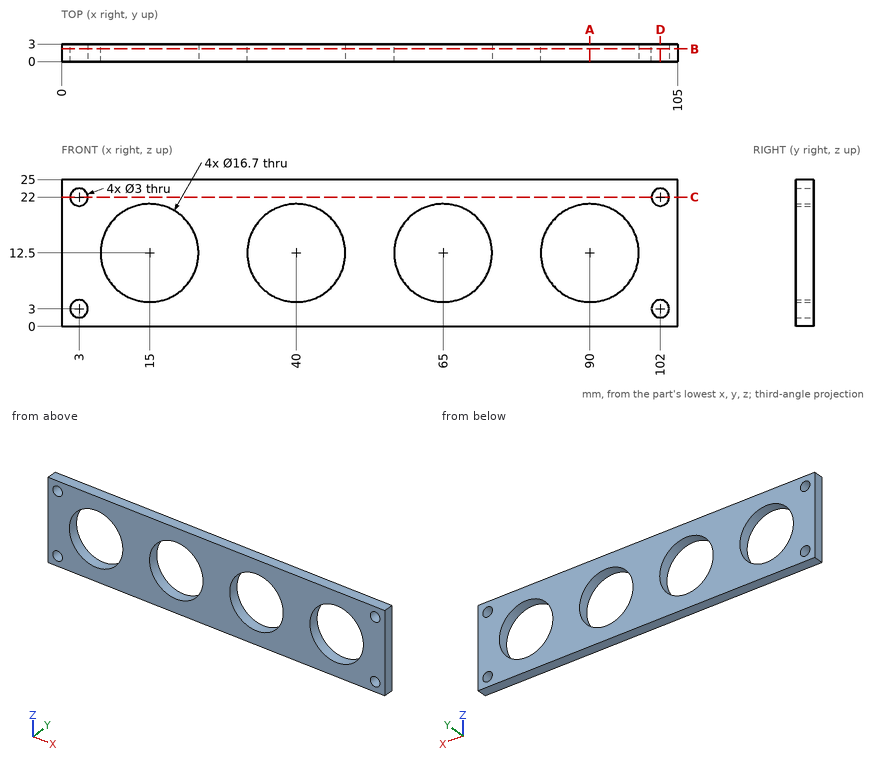
The drawing under review shows one solid part. Ordinate dimensions are in mm from its lowest x, y, z. Round coordinates to 2 decimals unless told otherwise and drop trailing zeros. Write each loop counter-clockwise with the first axis right and the second up, starting at its lowest first coordinate (ties: lowest second). Pieces come first, ordered by that corner, then holes. Notation, with made-up numbers: (4, 56) -> (28, 56) arc R8 cw to (28, 71) -> close; hole circle Ø7 at (67.25, 24). An arc over 180 degrees is marked (long way). One line per question, with ' | ' between items.
(1) Take a section at C-C, the plane z = 22. State the section outline as (x, y) points.
Result sheet:
outline: (0, 0) -> (1.5, 0) -> (1.5, 3) -> (0, 3) -> close; (4.5, 0) -> (100.5, 0) -> (100.5, 3) -> (4.5, 3) -> close; (103.5, 0) -> (105, 0) -> (105, 3) -> (103.5, 3) -> close
(2) Take a section at D-D, the plane x = 102. State the section outline as (y, z) points, and give its area (3 significant figures).
Result sheet:
outline: (0, 0) -> (3, 0) -> (3, 1.5) -> (0, 1.5) -> close; (0, 4.5) -> (3, 4.5) -> (3, 20.5) -> (0, 20.5) -> close; (0, 23.5) -> (3, 23.5) -> (3, 25) -> (0, 25) -> close | area: 57.0 mm2
(3) Insertion check: P1, Ø4, axis at x = 51.5, z = 7, coming from the -Y side; P2, Ø13.5, axis at x = 15, z = 12.5, coming from the +Y side. Each pin has a flat end and moves straight along its axis. Give the tip position at first contact, or say it passes through.
Result sheet:
P1: y = 0 | P2: through
(4) Take a section at B-B, the plane y = 2.15. State how many separate pieces and enclosed holes the cut face has, and give its area (3 significant figures).
Result sheet:
separate pieces: 1 | enclosed holes: 8 | area: 1,720 mm2
(5) Wall thickness on line 1 (X direction, y = 1.95, z = 2.75); line 2 (Z direction, x = 90, y = 2.2); line 3 (X direction, y = 1.6, z = 9.25): over which ranges is each line inside the solid? List them lowest first. Write a range as [from, to].
Result sheet:
line 1: [0, 1.52], [4.48, 100.52], [103.48, 105] | line 2: [0, 4.15], [20.85, 25] | line 3: [0, 7.31], [22.69, 32.31], [47.69, 57.31], [72.69, 82.31], [97.69, 105]
(6) Take a section at A-A, the plane x = 90. State the section outline as (y, z) points, and give its area (3 significant figures).
Result sheet:
outline: (0, 0) -> (3, 0) -> (3, 4.15) -> (0, 4.15) -> close; (0, 20.85) -> (3, 20.85) -> (3, 25) -> (0, 25) -> close | area: 24.9 mm2
